```python
from build123d import *

# Parameters (mm, degrees)
F0_W     = 72
F0_H     = 116
F0_R     = 2.5
F0_R_2   = 6
F2_DEPTH = 6
F1_W     = 72
F1_H     = 22
F1_R     = 3
F3_DEPTH = 6
F4_SIZE  = 2
F5_SIZE  = 2
F6_SIZE  = 2
F7_R     = 25
F7_R_2   = 2.5
F7_R_3   = 6
F8_DEPTH = 2


with BuildPart() as f2:
    # F0 (on Front) → F2 (new body)
    with BuildSketch(Plane.XZ):
        with Locations((0, 58)):
            Rectangle(F0_W, F0_H)
        with Locations((-17.75, 69.752033)):
            Circle(F0_R, mode=Mode.SUBTRACT)
        with Locations((17.75, 69.752033)):
            Circle(F0_R, mode=Mode.SUBTRACT)
        with Locations((0, 80)):
            Circle(F0_R_2, mode=Mode.SUBTRACT)
        with Locations((0, 100.495935)):
            Circle(F0_R, mode=Mode.SUBTRACT)
    extrude(amount=-F2_DEPTH)

    # F1 (on Top) → F3 (join)
    with BuildSketch(Plane.XY):
        with Locations((0, 11)):
            Rectangle(F1_W, F1_H)
        with Locations((-24.75, 15)):
            Circle(F1_R, mode=Mode.SUBTRACT)
        with Locations((24.75, 15)):
            Circle(F1_R, mode=Mode.SUBTRACT)
    extrude(amount=F3_DEPTH)

    # F4
    f4_edges = [f2.edges().sort_by_distance(p)[0] for p in [
        (0, 6, 6),
    ]]
    chamfer(f4_edges, length=F4_SIZE)

    # F5
    f5_edges = [f2.edges().sort_by_distance(p)[0] for p in [
        (0, 0, 0),
    ]]
    chamfer(f5_edges, length=F5_SIZE)

    # F6
    f6_edges = [f2.edges().sort_by_distance(p)[0] for p in [
        (-2.5, 0, 100.495935),
        (-20.25, 0, 69.752033),
        (15.25, 0, 69.752033),
    ]]
    chamfer(f6_edges, length=F6_SIZE)

    # F7 (on face) → F8 (cut)
    with BuildSketch(Plane(origin=(0, 6, 0), x_dir=(-1, 0, 0), z_dir=(0, 1, 0))):
        with Locations((0, 80)):
            Circle(F7_R)
        with Locations((-17.75, 69.752033)):
            Circle(F7_R_2, mode=Mode.SUBTRACT)
        with Locations((17.75, 69.752033)):
            Circle(F7_R_2, mode=Mode.SUBTRACT)
        with Locations((0, 80)):
            Circle(F7_R_3, mode=Mode.SUBTRACT)
        with Locations((0, 100.495935)):
            Circle(F7_R_2, mode=Mode.SUBTRACT)
    extrude(amount=-F8_DEPTH, mode=Mode.SUBTRACT)


solid = f2.part
```
Here's how the part is built. I have some questions about the finished solid (model axes, mm). A direction names the side the tool comes from. Give positions to 0.01 mm unless a question says otherwise; leave off trailing zeros. Order: outer loops, then holes, each group sorted by start corner. A loop starts at its lowest first (then second) coordinate and runs counter-clockwise, first axis right, second up. Notation, with made-up numbers: M 36.25,48.25 L 54.25,48.25 A19 ccw 54.25,85.25 Z; hole C 3,-32 d4. An arc over 180 degrees is marked long. Use a Markdown table: item, result. Add a question column.
1. Suppose I cut it at D-D (x = -17.75). List the corners of the cut face in (y, z) for me, and give its area (3 significant figures).
2. Suppose I cut it at B-B (x = 0). List the corners of the cut face in (y, z) for me.
3. For pin 1 Ø4 at (x, z) = (0, 100.5) entering from -Y; pin 2 Ø6.5 at (x, z) = (-17.75, 69.75) entering from -Y; pin 3 Ø3 at (x, y) = (27, 10) entering from +Z, each with a flat end and sliding along its axis, tell me the tip position at first contact or that it passes through.
4. Suppose I cut it at C-C (z = 80). List the corners of the cut face in (x, y) for me, and give its area (3 significant figures).
5. I need wall thicknesses on probe 1 along Y at (x, z) = (-24.75, 2.4); probe 2 along Z at (x, y) = (0, 5.5); probe 3 along X at (y, z) = (1, 80). Which ranges of each line are inside material? Lowest first, please. Write a range as from..to.
6. On a 3-axis mill with a long thin cutter (end or side, diameter ignored), from which of +Z, -Z, +X, -X, +Y, -Y can I reach the whole of each face in a straight line? I mean faces 1 (the cylindrical face through (-0.325, 2.986, 102.975)), 2 (the flat face through (-1, 6, 51)), 3 (the cylindrical face through (5.42, 5.014, 55.594)). Say none if no direction works.
7. Suppose I cut it at A-A (y = 15). List the corners of the cut face in (x, z) for me.
8. If we mould it in two halves opening along X, with no side actions, what happens to faces 4 (the flat face through (-1, 12, 0)), 5 (the flat face through (36, 4, 44)), 6 (the cylindrical face through (17.21, 2.99, 67.31))? For each: +X half, -X half, draft (parallel to the pull), parting line (faces both ways), or undercut.
Results list:
| question | item | result |
|---|---|---|
| 1 | outline | M 0,2 L 2,0 L 22,0 L 22,6 L 8,6 L 6,8 L 6,62.39 L 4,62.39 L 4,67.25 L 2,67.25 L 0,65.25 Z; M 0,74.25 L 2,72.25 L 4,72.25 L 4,97.61 L 6,97.61 L 6,116 L 0,116 Z |
| 1 | area | 698 mm² |
| 2 | outline | M 0,2 L 2,0 L 22,0 L 22,6 L 8,6 L 6,8 L 6,55 L 4,55 L 4,74 L 0,74 Z; M 0,86 L 4,86 L 4,98 L 2,98 L 0,96 Z; M 0,105 L 2,103 L 4,103 L 4,105 L 6,105 L 6,116 L 0,116 Z |
| 3 | pin 1 | passes through |
| 3 | pin 2 | stops at y = 1.25 |
| 3 | pin 3 | stops at z = 6 |
| 4 | outline | M -36,0 L -6,0 L -6,4 L -25,4 L -25,6 L -36,6 Z; M 6,0 L 36,0 L 36,6 L 25,6 L 25,4 L 6,4 Z |
| 4 | area | 284 mm² |
| 5 | probe 1 | y = 0..12, 18..22 |
| 5 | probe 2 | z = 0..55, 105..116 |
| 5 | probe 3 | x = -36..-6, 6..36 |
| 6 | face 1 | +Y, -Y |
| 6 | face 2 | +Z, +X, -X, +Y |
| 6 | face 3 | +Y |
| 7 | outline | M -36,0 L -27.75,0 L -27.75,6 L -36,6 Z; M -21.75,0 L 21.75,0 L 21.75,6 L -21.75,6 Z; M 27.75,0 L 36,0 L 36,6 L 27.75,6 Z |
| 8 | face 4 | draft |
| 8 | face 5 | +X half |
| 8 | face 6 | undercut |
